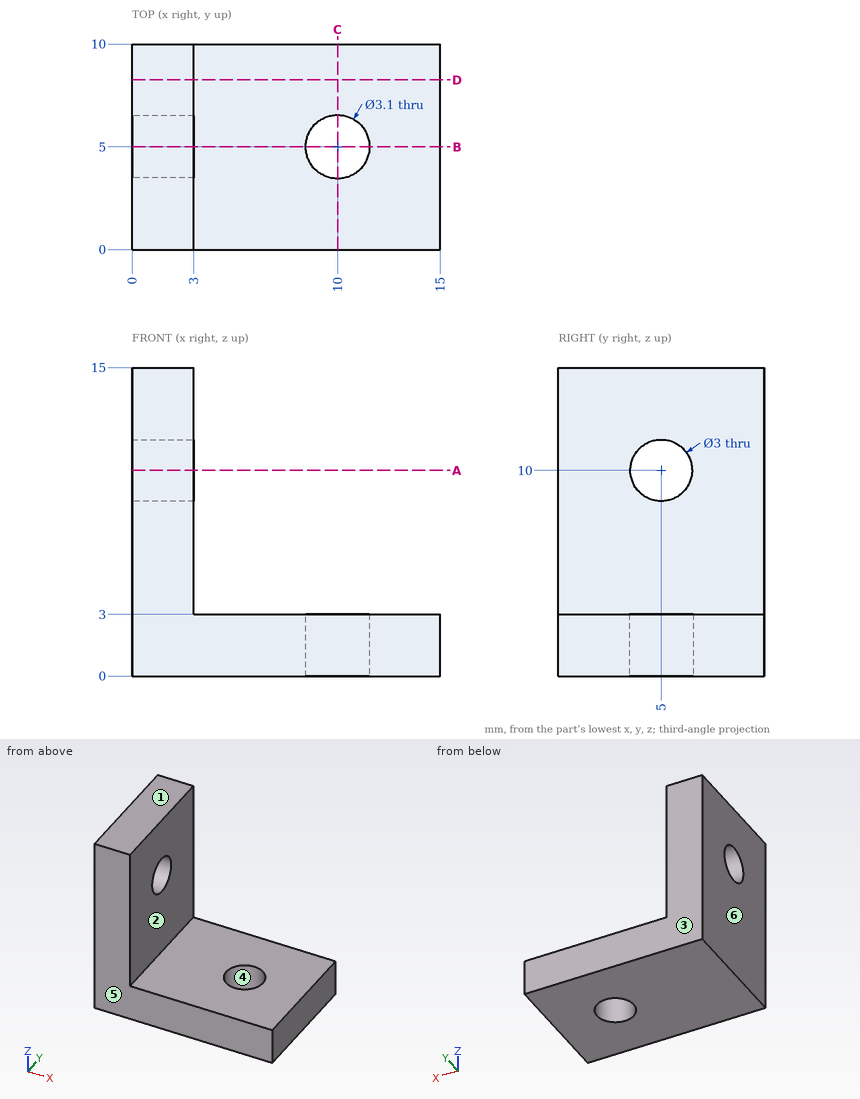
Could you check a few things on this drawing? It's one solid part, dimensions in mm from its lowest x, y, z. A direction names the side the tool comes from. Give positions to 0.01 mm unless a question says otherwise; leave off trailing zeros. Loops run counter-clockwise (first coordinate to the right, second up) from the corner with the lowest first, then second, coordinate; pieces in that order, holes last. Notation, with made-up numbers: (-6.75, -16) -> (18.25, -16) arc R26 cw to (18.25, 10) -> close; hole circle Ø2 at (53.25, 83.5). An arc over 180 degrees is marked (long way). Answer as CSV lines item,"result". Start each with the question number.
(1) If we section it at C-C on x = 10: Write out the boundary of the cut face in (y, z), then the cut area to 3 significant figures.
(2) I need wall thicknesses on probe 1 along Y at (x, z) = (2.4, 10); probe 2 along X at (y, z) = (4.75, 12). Which ranges of each line are inside material? Lowest first, please.
(3) Which directions (+Z, -Z, +X, -X, +Y, -Y) give clear straight access to the entire face, cutting with the end or side of a thin tool? Please do the marked faces 1 and 2.
(4) If we section it at D-D on y = 8.25: Write out the boundary of the cut face in (x, z).
(5) I'm going to push flat-ended pins straight in: pin 1 Ø6 at (x, z) = (8.5, 9) entering from +Y; pin 2 Ø2 at (x, y) = (9.5, 6) entering from +Z. Where does each tip first touch, or does it pass through?
(6) If we section it at B-B on y = 5: Write out the boundary of the cut face in (x, z), then the cut area to 3 significant figures.
(7) If we section it at A-A on z = 10: Write out the boundary of the cut face in (x, y).
(8) We'd pull the mould along Y, two halves only. Please class the marked faces 3, 4, 5 and 6: released by +Y, released by -Y, zero draft, split by the parting line, or undercut.
Computed:
1,outline,"(0, 0) -> (3.45, 0) -> (3.45, 3) -> (0, 3) -> close; (6.55, 0) -> (10, 0) -> (10, 3) -> (6.55, 3) -> close"
1,area,"20.7 mm2"
2,probe 1,"y = 0 to 3.5, 6.5 to 10"
2,probe 2,"x = 0 to 3"
3,face 1,"+Z, +X, -X, +Y, -Y"
3,face 2,"+Z, +X, +Y, -Y"
4,outline,"(0, 0) -> (15, 0) -> (15, 3) -> (3, 3) -> (3, 15) -> (0, 15) -> close"
5,pin 1,"passes through"
5,pin 2,"stops at z = 3"
6,outline,"(0, 0) -> (8.45, 0) -> (8.45, 3) -> (3, 3) -> (3, 8.5) -> (0, 8.5) -> close; (0, 11.5) -> (3, 11.5) -> (3, 15) -> (0, 15) -> close; (11.55, 0) -> (15, 0) -> (15, 3) -> (11.55, 3) -> close"
6,area,"62.7 mm2"
7,outline,"(0, 0) -> (3, 0) -> (3, 3.5) -> (0, 3.5) -> close; (0, 6.5) -> (3, 6.5) -> (3, 10) -> (0, 10) -> close"
8,face 3,"released by +Y"
8,face 4,"undercut"
8,face 5,"released by -Y"
8,face 6,"zero draft"
